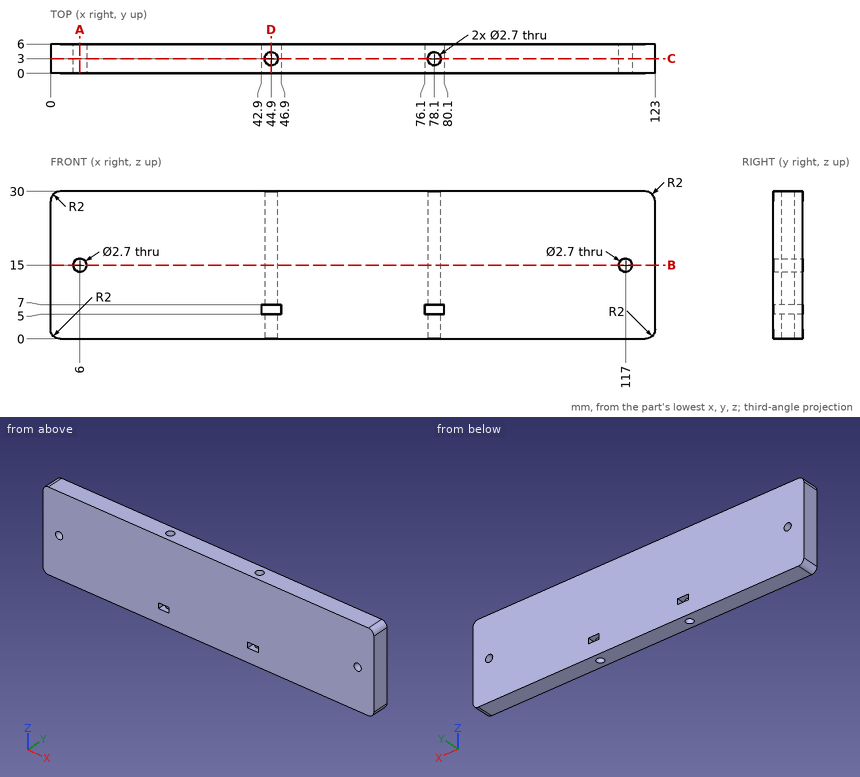
For this review, use the dimensioned drawing (mm, ordinates from the lowest corner) and the shaded views. Give positions to 0.01 mm unless a question says otherwise; leave off trailing zeros. Write each loop counter-clockwise with the first axis right and the second up, starting at its lowest first coordinate (ties: lowest second). Pieces come first, ordered by that corner, then holes. Notation, with made-up numbers: M -22,-39.75 L 36,-39.75 A18 cw 36,-12.75 Z; hole C 26.5,71 d2. An arc over 180 degrees is marked long. Answer as a JSON object with one key per item and string values. Group by question number.
Item 1: For pin 1 Ø2.5 at (x, y) = (78.1, 3) entering from -Z, flat-tipped, find the tip position at first contact; note if it passes through.
Item 2: For probe 1 along X at (y, z) = (3, 19); probe 2 along Y at (x, z) = (78.1, 1.9); probe 3 along Z at (x, y) = (6, 3.25), list the stretches that pass through material, from the lowest coordinate up. Write a range as [from, to].
Item 3: Consider section B-B on z = 15. Write out the cut boundary in (x, y).
Item 4: Consider section C-C on y = 3. Count the separate pieces of the cut face and the enclosed holes in it, plus the area to 3 significant figures.
Item 5: Consider section A-A on x = 6. Write out the cut boundary in (y, z), plus the area to 3 significant figures.
Item 6: Consider section D-D on x = 44.9. Write out the cut boundary in (y, z), plus the area to 3 significant figures.
Check result:
{
 "1": {"pin 1": "passes through"},
 "2": {"probe 1": "x = [0, 43.55], [46.25, 76.75], [79.45, 123]", "probe 2": "y = [0, 1.65], [4.35, 6]", "probe 3": "z = [0, 13.65], [16.35, 30]"},
 "3": {"outline": "M 0,0 L 4.65,0 L 4.65,6 L 0,6 Z; M 7.35,0 L 115.65,0 L 115.65,6 L 7.35,6 Z; M 118.35,0 L 123,0 L 123,6 L 118.35,6 Z; hole C 44.9,3 d2.7; hole C 78.1,3 d2.7"},
 "4": {"separate pieces": "3", "enclosed holes": "2", "area": "3,510 mm^2"},
 "5": {"outline": "M 0,0 L 6,0 L 6,13.65 L 0,13.65 Z; M 0,16.35 L 6,16.35 L 6,30 L 0,30 Z", "area": "164 mm^2"},
 "6": {"outline": "M 0,0 L 1.65,0 L 1.65,5 L 0,5 Z; M 0,7 L 1.65,7 L 1.65,30 L 0,30 Z; M 4.35,0 L 6,0 L 6,5 L 4.35,5 Z; M 4.35,7 L 6,7 L 6,30 L 4.35,30 Z", "area": "92.4 mm^2"}
}
